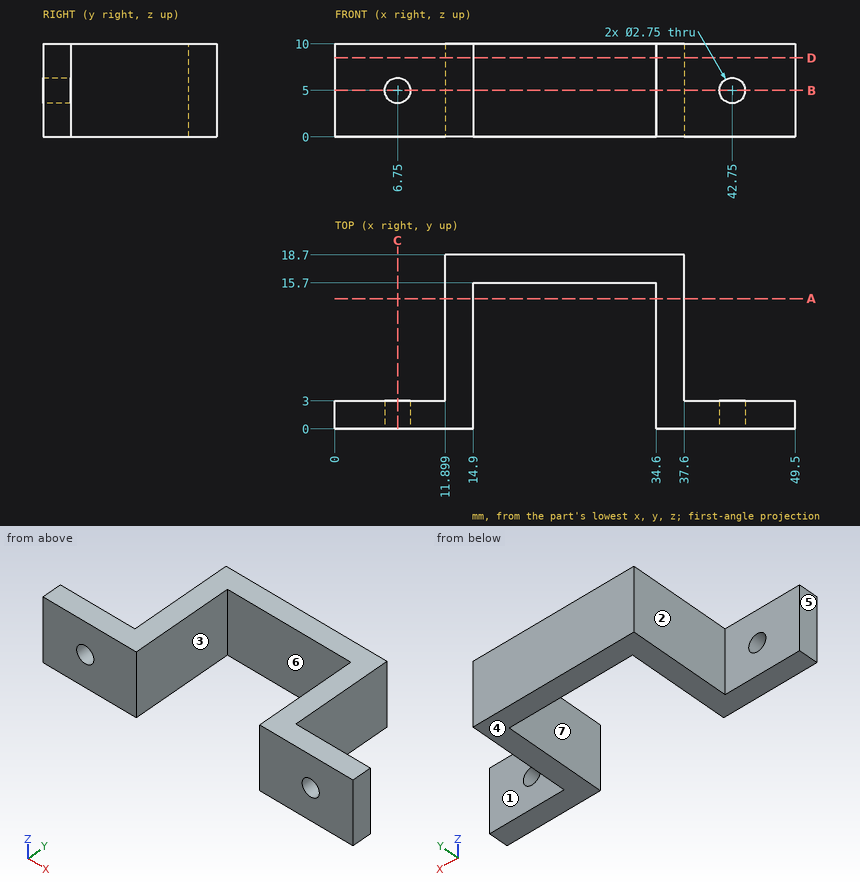
Job drawing, mm, ordinate dimensions from the low corner. One solid piece. A direction names the side the tool comes from. Give positions to 0.01 mm unless a question says otherwise; leave off trailing zeros. Loops run counter-clockwise (first coordinate to the right, second up) from the corner with the lowest first, then second, coordinate; pieces in that order, holes last.
Item 1: Which spindle directions (+Z, -Z, +X, -X, +Y, -Y) get a long thin tool onto all of the face, cutting with end or side? Do the marked faces 1, 2 and 3. Say none if no direction does.
Answers follow:
face 1: +Z, -Z, +X, +Y
face 2: +Z, -Z, -X, +Y
face 3: +Z, -Z, -Y
Item 2: Slice it at B-B, the plane z = 5. List the corners of the cut face in (x, y) (1 decimal), and give its area (3 significant figures).
Answers follow:
outline: (0, 0) - (5.4, 0) - (5.4, 3) - (0, 3) - close; (8.1, 0) - (14.9, 0) - (14.9, 15.7) - (34.6, 15.7) - (34.6, 0) - (41.4, 0) - (41.4, 3) - (37.6, 3) - (37.6, 18.7) - (11.9, 18.7) - (11.9, 3) - (8.1, 3) - close; (44.1, 0) - (49.5, 0) - (49.5, 3) - (44.1, 3) - close
area: 226 mm2
Item 3: Slice it at A-A, the plane y = 14. List the corners of the cut face in (x, z).
Answers follow:
outline: (11.9, 0) - (14.9, 0) - (14.9, 10) - (11.9, 10) - close; (34.6, 0) - (37.6, 0) - (37.6, 10) - (34.6, 10) - close
Item 4: Slice it at C-C, the plane x = 6.75. List the corners of the cut face in (y, z) (1 decimal).
Answers follow:
outline: (0, 0) - (3, 0) - (3, 3.6) - (0, 3.6) - close; (0, 6.4) - (3, 6.4) - (3, 10) - (0, 10) - close
Item 5: Pull direction X, two halves, no side cores. Call the marked faces 4, 5, 6 and 7: released by +X, released by -X, zero draft, split by the parting line, or undercut.
Answers follow:
face 4: zero draft
face 5: released by -X
face 6: undercut
face 7: undercut
Item 6: Drill centre lines: line 1 (X direction, y = 2.2, z = 5) (1 decimal); line 2 (X direction, y = 9, z = 4); line 3 (Y direction, x = 41, z = 4). Where is each one in solid material? Low to high.
Answers follow:
line 1: x = 0 to 5.4, 8.1 to 14.9, 34.6 to 41.4, 44.1 to 49.5
line 2: x = 11.9 to 14.9, 34.6 to 37.6
line 3: y = 0 to 3
Item 7: Flat gauge pins, fed straight in: pin 1 (5 mm diameter, centred on y = 14, z = 4.5, fed in from +X); pin 2 (3.5 mm diameter, centred on x = 6.75, z = 5, fed in from +Y); pin 3 (5 mm diameter, centred on y = 6.5, z = 4, fed in from -X); pin 4 (1.6 mm diameter, centred on x = 42.75, z = 5, fed in from -Y). Where does each tip first touch, or does it go through?
Answers follow:
pin 1: stops at x = 37.6
pin 2: stops at y = 3
pin 3: stops at x = 11.9
pin 4: passes through
Item 8: Slice it at D-D, the plane z = 8.5. List the corners of the cut face in (x, y).
Answers follow:
outline: (0, 0) - (14.9, 0) - (14.9, 15.7) - (34.6, 15.7) - (34.6, 0) - (49.5, 0) - (49.5, 3) - (37.6, 3) - (37.6, 18.7) - (11.9, 18.7) - (11.9, 3) - (0, 3) - close
